Source: three-view drawing plus pictorial views. Frame: mm from the lowest corner of the part. Give positions to 0.01 mm unless a question says otherwise; leave off trailing zeros. Loops run counter-clockwise (first coordinate to the right, second up) from the corner with the lowest first, then second, coordinate; pieces in that order, holes last. Notation, with made-up numbers: M 14,-19 L 21,-19 A15 ccw 21,-4 Z; hole C 19,-26.5 d4. An arc over 180 degrees is marked long. One line per item, written item: value. Start each with the question number.
(1) Section A-A on x = 80. Output: boundary loops of the cut face in (y, z).
(2) Section B-B on y = 50. Output: boundary loops of the cut face in (x, z), plus the area to 3 significant figures.
(3) Section C-C on z = 0.7. Output: boundary loops of the cut face in (x, y), plus the area to 3 significant figures.
(4) Ray query, line 1 along X through (y, z) = (140, 2.45); line 2 along Y through (x, z) = (15, 1.7); line 3 along Y through (x, z) = (80, 2.3). Return the intervals inside material, ascending. Write a range as from..to.
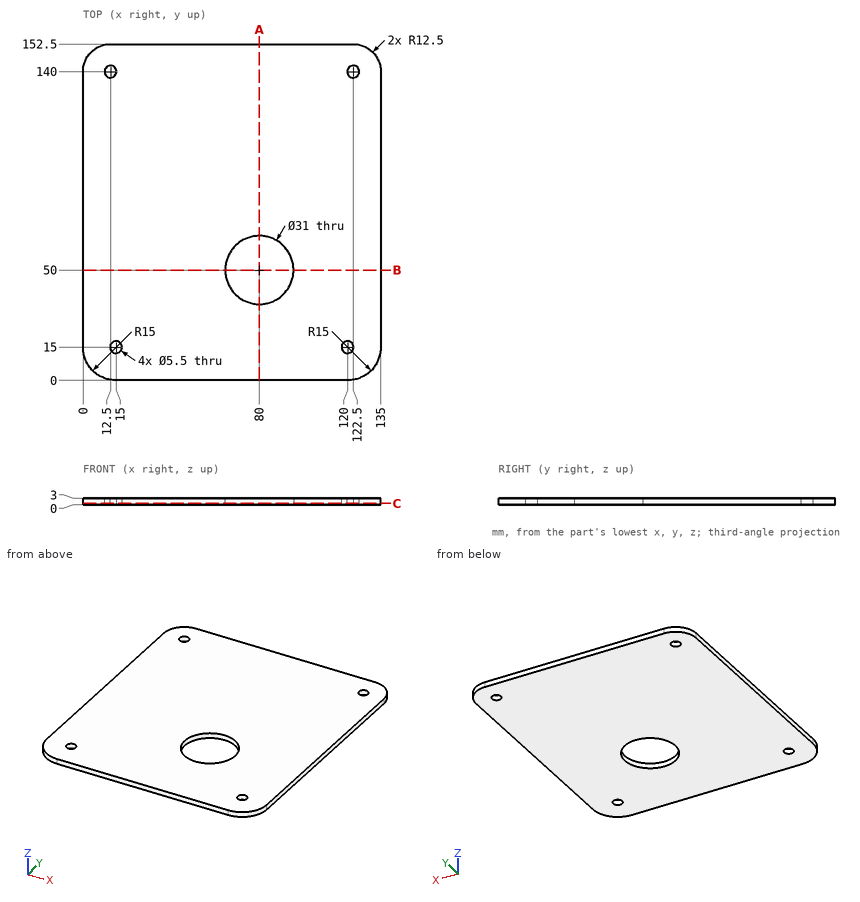
Output values:
1. outline: M 0,0 L 34.5,0 L 34.5,3 L 0,3 Z; M 65.5,0 L 152.5,0 L 152.5,3 L 65.5,3 Z
2. outline: M 0,0 L 64.5,0 L 64.5,3 L 0,3 Z; M 95.5,0 L 135,0 L 135,3 L 95.5,3 Z
2. area: 312 mm²
3. outline: M 0,15 A15 ccw 15,0 L 120,0 A15 ccw 135,15 L 135,140 A12.5 ccw 122.5,152.5 L 12.5,152.5 A12.5 ccw 0,140 Z; hole C 12.5,140 d5.5; hole C 15,15 d5.5; hole C 80,50 d31; hole C 120,15 d5.5; hole C 122.5,140 d5.5
3. area: 19,600 mm²
4. line 1: x = 0..9.75, 15.25..119.75, 125.25..135
4. line 2: y = 0..12.25, 17.75..138.85, 141.15..152.5
4. line 3: y = 0..34.5, 65.5..152.5
